Part model, mm, in its own coordinate system. Face numbers are marked on the shaded views. Give positions to 0.01 mm unless a question says otherwise; leave off trailing zeros. Order: outer loops, then holes, each group sorted by start corner. A loop starts at its lowest first (then second) coordinate and runs counter-clockwise, first axis right, second up.
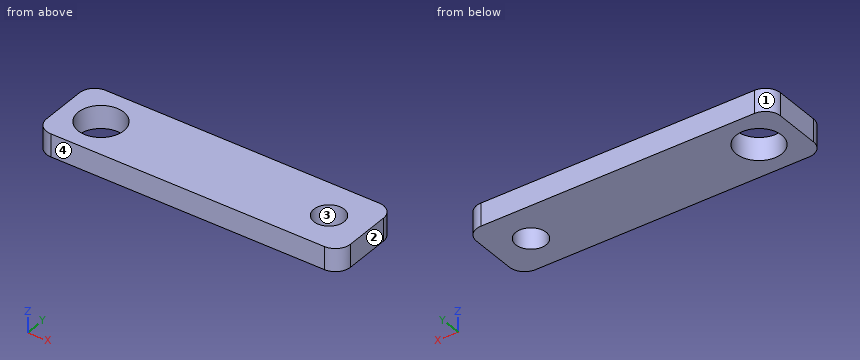
Autodesk Inventor part; units mm, degrees
ref_plane "YZ Plane" through (0, 0, 0) normal (1, 0, 0) x (0, 1, 0)
ref_plane "XZ Plane" through (0, 0, 0) normal (0, 1, 0) x (-1, 0, 0)
ref_plane "XY Plane" through (0, 0, 0) normal (0, 0, 1) x (1, 0, 0)
sketch "Эскиз1" plane through (0, 0, 0) normal (0, 0, 1) x (1, 0, 0)
  line L0 (-4.7967, -2.561) -> (35.2033, -2.561)
  line L1 (35.2033, -2.561) -> (35.2033, 7.439)
  line L2 (35.2033, 7.439) -> (-4.7967, 7.439)
  line L3 (-4.7967, 7.439) -> (-4.7967, -2.561)
  point P0 (0, 0)
  dimension "d0" = 10
  dimension "d1" = 40
extrude "Выдавливание1" add sketch "Эскиз1" along normal blind 3
sketch "Эскиз2" plane through (0, 0, 3) normal (0, 0, 1) x (1, 0, 0)
  line L0 (-4.7967, 7.439) -> (-4.7967, -2.561)
  circle A0 centre (0.2033, 2.439) radius 3
  circle A1 centre (30.2033, 2.439) radius 2
  line L1 (35.2033, -2.561) -> (35.2033, 7.439)
  point P0 (0, 0)
  point P1 (-4.7967, 2.439)
  dimension "d4" = 6
  dimension "d5" = 5
  dimension "d6" = 4
  dimension "d7" = 5
extrude "Выдавливание2" cut sketch "Эскиз2" against normal blind 10
fillet "Сопряжение1" radius 2 4 edges at (-4.7967, 7.439, 1.5) (-4.7967, -2.561, 1.5) (35.2033, -2.561, 1.5) (35.2033, 7.439, 1.5)
properties part number "лапка сервы"
Item 1: Band-saw the part on C-C on x = 1. List the corners of the cut face in (y, z).
Item 2: Band-saw the part on D-D on y = 3.5. List the corners of the cut face in (x, z), plus the area to 3 significant figures.
Item 3: Drill centre lines: probe 1 along X at (y, z) = (2.5, 1.1); probe 2 along X at (y, z) = (1.25, 1.35); probe 3 along X at (y, z) = (0, 1.65). Where is each one in solid material? Low to high.
Item 4: Pull direction Y, two halves, no side cores. Call the marked faces 1, 2, 3 and 4: released by +Y, released by -Y, zero draft, split by the parting line, or undercut.
Item 5: Band-saw the part on A-A on y = 2. List the corners of the cut face in (x, z), plus the area to 3 significant figures.
Item 6: Band-saw the part on B-B on z = 2.15. List the corners of the cut face in (x, y), plus the area to 3 significant figures.
Working result:
1. outline: (-2.56, 0) - (-0.45, 0) - (-0.45, 3) - (-2.56, 3) - close; (5.33, 0) - (7.44, 0) - (7.44, 3) - (5.33, 3) - close
2. outline: (-4.8, 0) - (-2.6, 0) - (-2.6, 3) - (-4.8, 3) - close; (3.01, 0) - (28.51, 0) - (28.51, 3) - (3.01, 3) - close; (31.9, 0) - (35.2, 0) - (35.2, 3) - (31.9, 3) - close
2. area: 93.0 mm2
3. probe 1: x = -4.8 to -2.8, 3.2 to 28.2, 32.2 to 35.2
3. probe 2: x = -4.8 to -2.55, 2.96 to 28.6, 31.81 to 35.2
3. probe 3: x = -4.8 to -1.54, 1.95 to 35.2
4. face 1: released by +Y
4. face 2: zero draft
4. face 3: undercut
4. face 4: released by -Y
5. outline: (-4.8, 0) - (-2.76, 0) - (-2.76, 3) - (-4.8, 3) - close; (3.17, 0) - (28.25, 0) - (28.25, 3) - (3.17, 3) - close; (32.15, 0) - (35.2, 0) - (35.2, 3) - (32.15, 3) - close
5. area: 90.5 mm2
6. outline: (-4.8, -0.56) arc R2 ccw to (-2.8, -2.56) - (33.2, -2.56) arc R2 ccw to (35.2, -0.56) - (35.2, 5.44) arc R2 ccw to (33.2, 7.44) - (-2.8, 7.44) arc R2 ccw to (-4.8, 5.44) - close; hole circle Ø6 at (0.2, 2.44); hole circle Ø4 at (30.2, 2.44)
6. area: 356 mm2
